from build123d import *

# Parameters (mm, degrees)
F0_R          = 12.7
F4_DEPTH      = 25.908
F5_DEPTH      = 14.732
F5_DEPTH_BACK = 0.5334
F6_DEPTH      = 51.816
F7_R          = 6.7567647924
F8_DEPTH      = 76.454
F10_DEPTH     = 115.57
F11_R         = 5.08


with BuildPart() as f4:
    # F0 (on Front) → F4 (new body, symmetric)
    with BuildSketch(Plane.XZ):
        with BuildLine():
            Line((182.4113020967, 0), (22.352, 0))
            ThreePointArc((22.352, 0), (-15.8052507731, 15.8052507731), (0, -22.352))
            Line((0, -22.352), (194.2084, -22.352))
            Line((194.2084, -22.352), (194.2084, -11.7970979033))
            ThreePointArc((194.2084, -11.7970979033), (190.7531100225, -3.4552899775), (182.4113020967, 0))
        make_face()
        Circle(F0_R, mode=Mode.SUBTRACT)
    extrude(amount=F4_DEPTH, both=True)

    # F3 (on offset) → F5 (join, two sides)
    with BuildSketch(Plane.XZ.offset(25.4)) as f5_sk:
        with BuildLine():
            ThreePointArc((131.8115741014, 31.148834154), (130.990690219, 14.4909643817), (122.7341517806, 0))
            Line((122.7341517806, 0), (148.645862937, 0))
            Line((148.645862937, 0), (148.645862937, 27.3769088089))
            ThreePointArc((148.645862937, 27.3769088089), (147.3251483028, 30.062921432), (144.5359289646, 31.148834154))
            Line((144.5359289646, 31.148834154), (131.8115741014, 31.148834154))
        make_face()
    extrude(amount=-F5_DEPTH)
    extrude(f5_sk.sketch, amount=F5_DEPTH_BACK)

    # F1 (on Top) → F6 (cut, symmetric)
    with BuildSketch(Plane.XY):
        Polygon((-22.3446302116, 11.6586), (-22.3446302116, 0), (-22.3446302116, -11.6587262601), (35.7894971967, -11.6587262601), (35.7894971967, 11.6586), align=None)
    extrude(amount=F6_DEPTH, both=True, mode=Mode.SUBTRACT)

    # F7 (on Top) → F8 (cut)
    with BuildSketch(Plane.XY):
        with Locations((153.7918448448, 7.6698409393)):
            Circle(F7_R)
    extrude(amount=-F8_DEPTH, mode=Mode.SUBTRACT)

    # F9 (on Front) → F10 (cut)
    with BuildSketch(Plane.XZ):
        Polygon((122.7312460542, -22.4210973829), (122.7312460542, 0), (96.7673584819, 0), (103.2488569617, -22.4210973829), align=None)
    extrude(amount=F10_DEPTH, mode=Mode.SUBTRACT)

    # F11
    f11_edges = [f4.edges().sort_by_distance(p)[0] for p in [
        (22.352, -18.783363, 0),
        (22.352, 18.7833, 0),
        (148.645863, -18.288, 0),
    ]]
    fillet(f11_edges, radius=F11_R)


solid = f4.part
Input: part model. Units: mm. Frame: model coordinates. A direction names the side the tool comes from. Coordinates: 2 decimals unless noted, no trailing zeros. Loops run counter-clockwise (first coordinate to the right, second up) from the corner with the lowest first, then second, coordinate; pieces in that order, holes last. Notation, with made-up numbers: (25.25, 58.25) -> (67.25, 58.25) arc R27 cw to (67.25, 97.25) -> close; hole circle Ø7 at (46.5, 32). An arc over 180 degrees is marked (long way). Write item = value, one per line. Start each with the question number.
Item 1: Cut plane B-B, the plane z = 17.5. Return loops of the section in (x, y), plus the area to 3 significant figures.
Item 2: First-contact query: P1, Ø12, axis at y = -22, z = 15.5, coming from the +X side; P2, Ø25, axis at x = 133, z = 13.5, coming from the +Y side; P3, Ø13.5, axis at x = 156.5, z = -11, coming from the -Y side. Flat tips, straight axial feed; report the tip coordinate or a pass-through.
Item 3: Cut plane C-C, the plane y = 17.5. Return loops of the section in (x, z), plus the area to 3 significant figures.
Item 4: Cut plane D-D, the plane x = 79.5. Return loops of the section in (y, z).
Item 5: Material intervals for line 1 (Z direction, x = 0, y = -15); line 2 (X direction, y = -21.5, z = -10); line 3 (X direction, y = 7, z = -12.5), sorted ascending.
Item 6: Reachability of faces 1 (the face through (23.8, -18.9, 1.1)), 2 (the face through (96, 0, -22.352)), 3 (the face through (147.36, -18.19, 30.03)), 4 (the face through (106, 5, 0)), 5 (the face through (131.056, -18.194, 14.717)) from +Z, -Z, +X, -X, +Y, -Y: full face, straight path, thin tool, end or side. Return the list, or none.
Item 7: Mould query, pull axis X, two halves, no side actions, for faces 6 (the face through (150.17, -18.39, 1.45)), 7 (the face through (141, -10.668, 16)), 8 (the face through (122.731, -13, -11)). Classes: pulls with the +X half, pulls with the -X half, needs draft (parallel to the pull), parting line crosses it, or undercut.
Ans:
q1.outline = (-13.91, -25.91) -> (13.91, -25.91) -> (13.91, -11.66) -> (-13.91, -11.66) -> close; (-13.91, 11.66) -> (13.91, 11.66) -> (13.91, 25.91) -> (-13.91, 25.91) -> close; (131.73, -25.93) -> (148.65, -25.93) -> (148.65, -10.67) -> (131.73, -10.67) -> close
q1.area = 1,050 mm²
q2.P1 = 148.65
q2.P2 = -10.67
q2.P3 = -25.91
q3.outline = (0, -22.35) -> (194.21, -22.35) -> (194.21, -11.8) arc R11.8 ccw to (182.41, 0) -> (26.96, 0) arc R5.08 cw to (21.97, 4.14) arc R22.35 ccw (long way) to start; hole circle Ø25.4 at (0, 0)
q3.area = 4,990 mm²
q4.outline = (-25.91, -22.35) -> (25.91, -22.35) -> (25.91, 0) -> (-25.91, 0) -> close
q5.line_1 = -22.35 to -12.7, 12.7 to 22.35
q5.line_2 = -19.99 to -7.83, 7.83 to 99.66, 122.73 to 194.07
q5.line_3 = 35.79 to 147.07, 160.52 to 194.21
q6.face_1 = +Z, +Y, -Y
q6.face_2 = -Z, +X, -X, +Y, -Y
q6.face_3 = +Z, +X, +Y, -Y
q6.face_4 = +Z, +Y
q6.face_5 = +Y, -Y
q7.face_6 = pulls with the +X half
q7.face_7 = needs draft
q7.face_8 = undercut
